For this review, take the finished solid that the model builds, in its own axes (mm). A direction names the side the tool comes from. Give positions to 0.01 mm unless a question says otherwise; leave off trailing zeros. Write each loop counter-clockwise with the first axis right and the second up, starting at its lowest first coordinate (ties: lowest second). Pieces come first, ordered by that corner, then holes.
Q1. We need section C-C (z = -18.5). Write out the cut boundary in (x, y), then the cut area to 3 significant figures.
Q2. Insertion check: P1, Ø2, axis at x = 36, z = -71, coming from the -Y side; P2, Ø1.6, axis at y = -4.825, z = -65.475, coming from the -X side (3 decimals); P3, Ø2.5, axis at y = -4.825, z = -9.525, coming from the +X side (3 decimals). Each pin has a flat end and moves straight along its axis. Give the tip position at first contact, or say it passes through.
Q3. We need section A-A (z = -71). Write out the cut boundary in (x, y), then the cut area to 3 significant figures.
Q4. For line 1 (X direction, y = -5.25, z = -71); line 2 (Z direction, x = 92, y = -7.25); line 3 (Z direction, x = 91.5, y = -4.5), list the stretches that pass through material, from the lowest coordinate up.
Q5. Machinability: for faces 5 (the cylindrical face through (91.304, -3.484, -65.299)), 6 (the cylindrical face through (4.696, -4.766, -66.826)), 7 (the flat face through (49, -1.65, -38)), which of the approach directions +Z, -Z, +X, -X, +Y, -Y give a long, thin tool a straight path to every point of the face, cutting with its end or side? Answer none if there is none.
Q6. We need section B-B (x = 46.25). Write out the cut boundary in (y, z), then the cut area to 3 significant figures.
Q7. Mouldability with a two-part tool opening along X and no side actions: class faces 1 (the flat face through (9.525, -5, -65)), 2 (the cylindrical face through (80.37, -4.87, -13.93)), 3 (the flat face through (49, -5, 0)), 4 (the flat face through (86.475, -5, -10)) as released by +X, released by -X, zero draft, split by the parting line, or undercut.
```python
from build123d import *

# Parameters (mm, degrees)
SKETCH1_W           = 96
SKETCH1_H           = 75
BOSS_EXTRUDE1_DEPTH = 6.35
SKETCH2_R           = 1.63195
CUT_EXTRUDE1_DEPTH  = 6.35
SKETCH3_R           = 1.35255
CUT_EXTRUDE2_DEPTH  = 9.525
SKETCH4_R           = 1.35255
CUT_EXTRUDE3_DEPTH  = 9.525


with BuildPart() as part:
    # Sketch1 → Boss-Extrude1 (new body)
    with BuildSketch(Plane(origin=(0, -8, 0), x_dir=(-1, 0, 0), z_dir=(0, -1, 0))):
        with Locations((-48, 37.5)):
            Rectangle(SKETCH1_W, SKETCH1_H)
    extrude(amount=-BOSS_EXTRUDE1_DEPTH)

    # Sketch2 → Cut-Extrude1 (cut)
    with BuildSketch(Plane.XZ.offset(8)):
        with Locations((36, -71)):
            Circle(SKETCH2_R)
        with Locations((46.25, -18.5)):
            Circle(SKETCH2_R)
        with Locations((82, -14)):
            Circle(SKETCH2_R)
        with Locations((92, -71)):
            Circle(SKETCH2_R)
    extrude(amount=-CUT_EXTRUDE1_DEPTH, mode=Mode.SUBTRACT)

    # Sketch3 → Cut-Extrude2 (cut)
    with BuildSketch(Plane.ZY):
        with Locations((-65.475, -4.825)):
            Circle(SKETCH3_R)
        with Locations((-9.525, -4.825)):
            Circle(SKETCH3_R)
    extrude(amount=-CUT_EXTRUDE2_DEPTH, mode=Mode.SUBTRACT)

    # Sketch4 → Cut-Extrude3 (cut)
    with BuildSketch(Plane(origin=(96, 0, 0), x_dir=(0, 0, -1), z_dir=(1, 0, 0))):
        with Locations((65.475, -4.825)):
            Circle(SKETCH4_R)
        with Locations((9.525, -4.825)):
            Circle(SKETCH4_R)
    extrude(amount=-CUT_EXTRUDE3_DEPTH, mode=Mode.SUBTRACT)


solid = part.part
```
Computed:
1. outline: (0, -8) - (44.62, -8) - (44.62, -1.65) - (0, -1.65) - close; (47.88, -8) - (96, -8) - (96, -1.65) - (47.88, -1.65) - close
1. area: 589 mm2
2. P1: passes through
2. P2: stops at x = 9.525
2. P3: stops at x = 86.475
3. outline: (0, -8) - (34.37, -8) - (34.37, -1.65) - (0, -1.65) - close; (37.63, -8) - (90.37, -8) - (90.37, -1.65) - (37.63, -1.65) - close; (93.63, -8) - (96, -8) - (96, -1.65) - (93.63, -1.65) - close
3. area: 568 mm2
4. line 1: x = 0 to 34.37, 37.63 to 90.37, 93.63 to 96
4. line 2: z = -75 to -72.63, -69.37 to 0
4. line 3: z = -75 to -72.55, -69.45 to -66.79, -64.16 to -10.84, -8.21 to 0
5. face 5: +X
5. face 6: -X
5. face 7: +Z, -Z, +X, -X, +Y
6. outline: (-8, -75) - (-1.65, -75) - (-1.65, -20.13) - (-8, -20.13) - close; (-8, -16.87) - (-1.65, -16.87) - (-1.65, 0) - (-8, 0) - close
6. area: 456 mm2
7. face 1: released by -X
7. face 2: undercut
7. face 3: zero draft
7. face 4: released by +X
